Autodesk Inventor part; units mm, degrees
ref_plane "YZ Plane" through (0, 0, 0) normal (1, 0, 0) x (0, 1, 0)
ref_plane "XZ Plane" through (0, 0, 0) normal (0, 1, 0) x (-1, 0, 0)
ref_plane "XY Plane" through (0, 0, 0) normal (0, 0, 1) x (1, 0, 0)
ref_plane "Work Plane1" through (368.3, -368.3, 4.7625) normal (0, 0, 1) x (0, -1, 0)
sketch "Sketch1" plane through (368.3, -368.3, 4.7625) normal (0, 0, 1) x (0, -1, 0)
  spline S0 degree 3 number of poles 884
  arc A0 (-72.2824, -174.5174) -> (-43.815, -186.309) centre (-43.815, -146.05) ccw
  line L0 (-43.815, -186.309) -> (12.7, -186.309)
  line L1 (-174.5174, -72.2824) -> (-72.2824, -174.5174)
  arc A1 (-186.309, -43.815) -> (-174.5174, -72.2824) centre (-146.05, -43.815) ccw
  line L2 (-186.309, 12.7) -> (-186.309, -43.815)
  line L3 (-88.9, 10.16) -> (-647.7, 10.16)
  line L4 (10.16, -647.7) -> (10.16, -88.9)
  circle A2 centre (-43.815, -146.05) radius 31.1151
  circle A3 centre (-146.05, -43.815) radius 31.115
  line L5 (0, 0) -> (-123.3999, -123.3999) construction
  line L6 (0, -186.309) -> (0, 0) construction
  line L7 (0, 0) -> (-186.309, 0) construction
  spline S1 degree 3 number of poles 404 construction
  circle A4 centre (-53.9492, -53.9495) radius 55.5504
  line L8 (12.319, -147.6375) -> (12.319, -128.3493)
  line L9 (12.319, -125.6507) -> (12.319, -102.9776)
  line L10 (12.319, -748.919) -> (12.319, 12.7)
  line L11 (0, 12.319) -> (-53.975, 12.319)
  line L12 (-61.0927, 12.319) -> (-100.199, 12.319)
  line L13 (-147.6375, 12.319) -> (0, 12.319)
  arc A5 (12.319, 0) -> (0, 12.319) centre (0, 0) ccw
  arc A6 (-147.6375, 12.319) -> (-153.1614, 10.462) centre (-147.6375, 3.175) ccw
  arc A7 (-147.6375, 12.319) -> (-156.7815, 3.175) centre (-147.6375, 3.175) ccw
  line L14 (-156.7815, 3.175) -> (-156.7815, -3.175)
  arc A8 (-156.7815, -3.175) -> (-154.0017, -9.7408) centre (-147.6375, -3.175) ccw
  arc A9 (-156.7815, -3.175) -> (-147.6375, -12.319) centre (-147.6375, -3.175) ccw
  line L15 (-147.6375, -12.7) -> (-147.6375, -12.319)
  arc A10 (10.462, -153.1614) -> (12.319, -147.6375) centre (3.175, -147.6375) ccw
  arc A11 (3.175, -156.7815) -> (12.319, -147.6375) centre (3.175, -147.6375) ccw
  line L16 (-3.175, -156.7815) -> (3.175, -156.7815)
  arc A12 (-9.7408, -154.0017) -> (-3.175, -156.7815) centre (-3.175, -147.6375) ccw
  arc A13 (-12.319, -147.6375) -> (-3.175, -156.7815) centre (-3.175, -147.6375) ccw
  line L17 (-12.319, -147.6375) -> (-12.7, -147.6375)
  arc A14 (-175.7313, 0.0762) -> (-179.8687, 0.0762) centre (-177.8, 0) ccw
  arc A15 (-179.8687, -0.0762) -> (-175.7313, -0.0762) centre (-177.8, 0) ccw
  arc A16 (-0.0762, -175.7313) -> (-0.0762, -179.8687) centre (0, -177.8) ccw
  arc A17 (0.0762, -179.8687) -> (0.0762, -175.7313) centre (0, -177.8) ccw
  line L18 (-147.6375, 12.319) -> (-186.309, 12.319)
  line L19 (-147.6375, 12.319) -> (0, 12.319)
  line L20 (-186.309, 12.319) -> (-186.309, -43.815)
  line L21 (12.319, -186.309) -> (12.319, 0)
  line L22 (-174.5174, -72.2824) -> (-72.2824, -174.5174)
  line L23 (12.319, -186.309) -> (-43.815, -186.309)
  arc A18 (-72.2824, -174.5174) -> (-43.815, -186.309) centre (-43.815, -146.05) ccw
  arc A19 (-186.309, -43.815) -> (-174.5174, -72.2824) centre (-146.05, -43.815) ccw
  arc A20 (12.319, 0) -> (-0.0762, 12.319) centre (-0.0004, -0.0002) ccw
  circle A21 centre (-0.0004, -0.0002) radius 1.8977
  circle A22 centre (-177.8, 0) radius 2.0701
  circle A23 centre (0, -177.8) radius 2.0701
  point P0 (-368.3, -368.3)
  point P1 (-153.5386, 10.16)
  point P2 (-186.309, 10.16)
  point P3 (10.16, -186.309)
  point P4 (10.16, -153.5386)
  point P5 (7.669, 9.6408)
  point P6 (-179.8687, -0.0762)
  point P7 (-179.8687, 0.0762)
  point P8 (-175.7313, 0.0762)
  point P9 (-175.7313, -0.0762)
  point P10 (0.0762, -179.8687)
  point P11 (-0.0762, -179.8687)
  point P12 (-0.0762, -175.7313)
  point P13 (0.0762, -175.7313)
extrude "Extrusion1" add sketch "Sketch1" along normal blind 3.175 contours L1 A1 L2 L3 A7 A6 L13 L12 L11 A5 L10 L9 L8 A10 A11 L4 L0 A0
sketch "Sketch2" plane through (368.3, -368.3, 4.7625) normal (0, 0, -1) x (-1, 0, 0)
  circle A0 centre (177.8, 0) radius 2.0701
  circle A1 centre (177.8, 0) radius 2.0701
  circle A2 centre (0, 177.8) radius 2.0701
  circle A3 centre (0, 177.8) radius 2.0701
  circle A4 centre (177.8, 0) radius 2.54
  circle A5 centre (0, 177.8) radius 2.54
  point P0 (368.3, 368.3)
  dimension "d2" = 5.08
  dimension "d3" = 5.08
extrude "Extrusion2" add sketch "Sketch2" along normal blind 7.9502
properties part number "swerve protector"
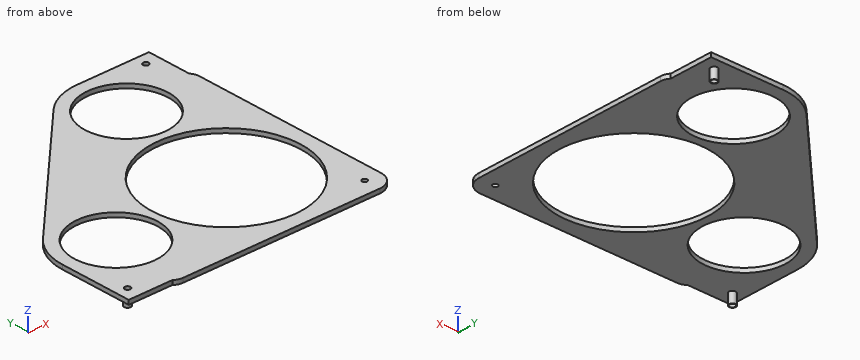
Geometry: final body of the model. Coordinates: model frame, mm. Coordinates: 2 decimals unless noted, no trailing zeros. Order: outer loops, then holes, each group sorted by start corner. A loop starts at its lowest first (then second) coordinate and runs counter-clockwise, first axis right, second up. Notation, with made-up numbers: M -20.5,85.25 L 16.5,85.25 A22 cw 16.5,113.25 Z; hole C 52,2 d4. An arc over 180 degrees is marked long. One line per question, with ' | ' between items. Start each with the question number.
Item 1: Cut plane A-A, the plane z = 0. Return the cut outline in (x, y).
Item 2: Cut plane C-C, the plane x = 361.5. Return the cut outline in (y, z).
Item 3: Cut plane D-D, the plane y = -317.5. Return the cut outline in (x, z), then the cut area to 3 significant figures.
Item 4: Ray query, probe 1 along X at (y, z) = (-368.3, 4); probe 2 along X at (y, z) = (-190.5, -0.25); probe 3 along X at (y, z) = (-340, 5.25). Return the intervals inside material, ascending. Write a range as [from, to].
Item 5: Pin query (flat end, axial travel): pin 1 Ø5 at (x, y) = (368.3, -368.3) entering from +Z; pin 2 Ø5 at (y, z) = (-264, 6.5) entering from -X; pin 3 Ø3.5 at (y, z) = (-195.5, 6) entering from +X; pin 4 Ø1 at (x, z) = (239, 6.5) entering from +Y. Return the tip coordinate at first contact, or that it passes through.
Item 6: Cut plane B-B, the plane y = -283. Return the cut outline in (x, z), then the cut area to 3 significant figures.
A:
1) outline: C 190.5,-368.3 d5.08; C 368.3,-190.5 d5.08; hole C 190.5,-368.3 d4.14; hole C 368.3,-190.5 d4.14
2) outline: M -380.62,4.76 L -343.72,4.76 L -343.72,7.94 L -380.62,7.94 Z; M -284.98,4.76 L -181.99,4.76 L -181.99,7.94 L -284.98,7.94 Z
3) outline: M 182.6,4.76 L 191.93,4.76 L 191.93,7.94 L 182.6,7.94 Z; M 252.57,4.76 L 258.89,4.76 L 258.89,7.94 L 252.57,7.94 Z; M 369.81,4.76 L 380.62,4.76 L 380.62,7.94 L 369.81,7.94 Z | area: 84.0 mm2
4) probe 1: x = [187.96, 188.43], [192.57, 193.04] | probe 2: x = [365.76, 366.23], [370.37, 370.84] | probe 3: x = [181.99, 195.28], [249.22, 265.08], [363.62, 380.62]
5) pin 1: stops at z = 7.94 | pin 2: stops at x = 223.3 | pin 3: stops at x = 378.46 | pin 4: stops at y = -250.3
6) outline: M 206.8,4.76 L 268.49,4.76 L 268.49,7.94 L 206.8,7.94 Z; M 360.21,4.76 L 380.62,4.76 L 380.62,7.94 L 360.21,7.94 Z | area: 261 mm2
